The model under review builds one solid part; all positions refer to its coordinate system, in mm. Face numbers are marked on the shaded views. A direction names the side the tool comes from. Round coordinates to 2 decimals unless told otherwise and drop trailing zeros. Write each loop counter-clockwise with the first axis right and the second up, starting at its lowest first coordinate (ties: lowest second). Pieces come first, ordered by that corner, then holes. Notation, with made-up numbers: (38, -28.75) -> (46, -28.75) arc R21 ccw to (46, -3.75) -> close; hole circle Ø6 at (83, -38). An arc over 180 degrees is marked (long way). Answer as a JSON object with one key per item and string values. Group by question number.
1) We need section C-C, the plane x = 3. Write out the cut boundary in (y, z).
2) Insertion check: pin 1 Ø6 at (x, z) = (0, 0) entering from +Y; pin 2 Ø1 at (y, z) = (0, -2.5) entering from -X; pin 3 Ø1 at (x, z) = (2.5, -3) entering from +Y; pin 4 Ø1.5 at (x, y) = (1, -0.5) entering from -Z. Each pin has a flat end and moves straight along its axis. Give the tip position at first contact, or say it passes through.
3) Machinability: for the marked faces 1 and 2, which of the approach directions +Z, -Z, +X, -X, +Y, -Y give a long, thin tool a straight path to every point of the face, cutting with its end or side? Answer none if there is none.
4) We need section A-A, the plane x = -3.25. Write out the cut boundary in (y, z), then the cut area to 3 significant figures.
5) Mouldability with a two-part tool opening along X and no side actions: class the marked faces 3 and 4 as pulls with the +X half, pulls with the -X half, needs draft (parallel to the pull), parting line crosses it, or undercut.
6) To check wall thickness, follow probe 1 along X at (y, z) = (0.1, 0); probe 2 along X at (y, z) = (1.95, 0); probe 3 along Y at (x, z) = (2.75, 0.5). State the ranges of each line that lie inside material, in increasing order. Write a range as [from, to].
7) We need section B-B, the plane y = -1.6. Write out the cut boundary in (x, z), then the cut area to 3 significant figures.
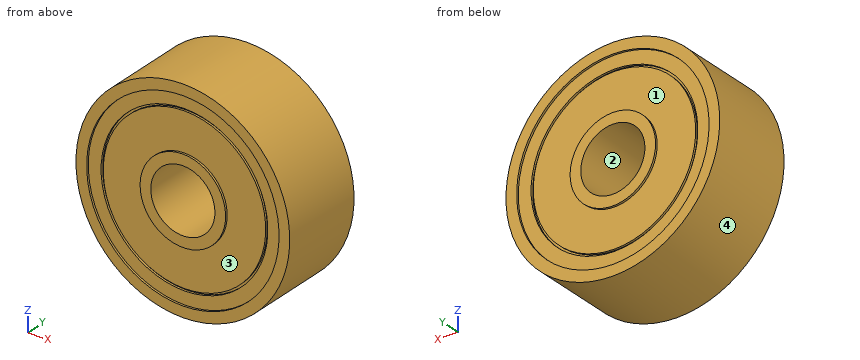
from build123d import *

# Parameters (mm, degrees)
SKETCH_1_R          = 5
SKETCH_1_R_2        = 1.5
EXTRUDE_1_DEPTH     = 2
SKETCH_2_R          = 4.5
SKETCH_2_R_2        = 2
CUT_EXTRUDE_1_DEPTH = 0.1
SKETCH_4_R          = 3.9
SKETCH_4_R_2        = 3.8
CUT_EXTRUDE_2_DEPTH = 0.1


with BuildPart() as part:
    # Эскиз1 → Бобышка-Вытянуть1 (new, symmetric)
    with BuildSketch(Plane(origin=(0, 0, 0), x_dir=(1, 0, 0), z_dir=(0, 1, 0))):
        with Locations(Location((0, 0, 0), (0, 0, 270))):
            Circle(SKETCH_1_R)
        with Locations(Location((0, 0, 0), (0, 0, 270))):
            Circle(SKETCH_1_R_2, mode=Mode.SUBTRACT)
    extrude(amount=EXTRUDE_1_DEPTH, both=True)

    # Эскиз2 → Вырез-Вытянуть1 (cut)
    with BuildSketch(Plane(origin=(0, 2, 0), x_dir=(1, 0, 0), z_dir=(0, 1, 0))):
        with Locations(Location((0, 0, 0), (0, 0, 270))):
            Circle(SKETCH_2_R)
        with Locations(Location((0, 0, 0), (0, 0, 270))):
            Circle(SKETCH_2_R_2, mode=Mode.SUBTRACT)
    cut_extrude_1 = extrude(amount=-CUT_EXTRUDE_1_DEPTH, mode=Mode.SUBTRACT)

    # Эскиз4 → Вырез-Вытянуть2 (cut)
    with BuildSketch(Plane(origin=(0, 1.9, 0), x_dir=(1, 0, 0), z_dir=(0, 1, 0))):
        with Locations(Location((0, 0, 0), (0, 0, 270))):
            Circle(SKETCH_4_R)
        with Locations(Location((0, 0, 0), (0, 0, 270))):
            Circle(SKETCH_4_R_2, mode=Mode.SUBTRACT)
    cut_extrude_2 = extrude(amount=-CUT_EXTRUDE_2_DEPTH, mode=Mode.SUBTRACT)

    # Зеркальное отражение1: Вырез-Вытянуть1, Вырез-Вытянуть2 across plane
    add(cut_extrude_1.mirror(Plane.ZX), mode=Mode.SUBTRACT)
    add(cut_extrude_2.mirror(Plane.ZX), mode=Mode.SUBTRACT)


solid = part.part
Here are the results:
{
 "1": {"outline": "(-2, -4) -> (2, -4) -> (2, -3.35) -> (1.9, -3.35) -> (1.9, -2.49) -> (1.8, -2.49) -> (1.8, -2.33) -> (1.9, -2.33) -> (1.9, 2.33) -> (1.8, 2.33) -> (1.8, 2.49) -> (1.9, 2.49) -> (1.9, 3.35) -> (2, 3.35) -> (2, 4) -> (-2, 4) -> (-2, 3.35) -> (-1.9, 3.35) -> (-1.9, 2.49) -> (-1.8, 2.49) -> (-1.8, 2.33) -> (-1.9, 2.33) -> (-1.9, -2.33) -> (-1.8, -2.33) -> (-1.8, -2.49) -> (-1.9, -2.49) -> (-1.9, -3.35) -> (-2, -3.35) -> close"},
 "2": {"pin 1": "stops at y = 2", "pin 2": "stops at x = -4.58", "pin 3": "stops at y = 1.9", "pin 4": "stops at z = -4.99"},
 "3": {"face 1": "+Y", "face 2": "+Y, -Y"},
 "4": {"outline": "(-2, -3.8) -> (2, -3.8) -> (2, -3.11) -> (1.9, -3.11) -> (1.9, -2.16) -> (1.8, -2.16) -> (1.8, -1.97) -> (1.9, -1.97) -> (1.9, 1.97) -> (1.8, 1.97) -> (1.8, 2.16) -> (1.9, 2.16) -> (1.9, 3.11) -> (2, 3.11) -> (2, 3.8) -> (-2, 3.8) -> (-2, 3.11) -> (-1.9, 3.11) -> (-1.9, 2.16) -> (-1.8, 2.16) -> (-1.8, 1.97) -> (-1.9, 1.97) -> (-1.9, -1.97) -> (-1.8, -1.97) -> (-1.8, -2.16) -> (-1.9, -2.16) -> (-1.9, -3.11) -> (-2, -3.11) -> close", "area": "29.1 mm^2"},
 "5": {"face 3": "undercut", "face 4": "parting line crosses it"},
 "6": {"probe 1": "x = [-5, -1.5], [1.5, 5]", "probe 2": "x = [-5, -4.5], [-2, -1.5], [1.5, 2], [4.5, 5]", "probe 3": "y = [-1.9, 1.9]"},
 "7": {"outline": "circle Ø10 at (0, 0); hole circle Ø3 at (0, 0)", "area": "71.5 mm^2"}
}
